The model under review builds one solid part; all positions refer to its coordinate system, in mm. A direction names the side the tool comes from. Coordinates: 2 decimals unless noted, no trailing zeros. Loops run counter-clockwise (first coordinate to the right, second up) from the corner with the lowest first, then second, coordinate; pieces in that order, holes last. Notation, with made-up numbers: M -27,-24.5 L 12,-24.5 A22 ccw 12,-14.5 Z; hole C 76,4.25 d7. An arc over 180 degrees is marked long. Use CSV: the item, a comma, the result in double quotes. Start each with the question number.
from build123d import *

# Parameters (mm, degrees)
SKETCH1_R           = 2.286
SKETCH1_R_2         = 1.27
BOSS_EXTRUDE1_DEPTH = 3.048
BOSS_EXTRUDE2_START = -3.048
BOSS_EXTRUDE2_DEPTH = 3.048
CIRPATTERN2_COUNT   = 18
BOSS_EXTRUDE3_START = 2.54
SKETCH3_R           = 1.75
SKETCH3_R_2         = 1.27
BOSS_EXTRUDE3_DEPTH = 2.54


with BuildPart() as part:
    # Sketch1 → Boss-Extrude1 (new body)
    with BuildSketch(Plane(origin=(0, 0, 0), x_dir=(1, 0, 0), z_dir=(0, 1, 0))):
        with Locations(Location((0, 0, 0), (0, 0, 90))):
            Circle(SKETCH1_R)
        with Locations(Location((0, 0, 0), (0, 0, 90))):
            Circle(SKETCH1_R_2, mode=Mode.SUBTRACT)
    extrude(amount=BOSS_EXTRUDE1_DEPTH)

    # Sketch2 → Boss-Extrude2 (add)
    with BuildSketch(Plane(origin=(0, 3.048, 0), x_dir=(1, 0, 0), z_dir=(0, 1, 0)).offset(BOSS_EXTRUDE2_START)):
        with BuildLine():
            Line((-0.127, 2.794), (0.127, 2.794))
            Line((0.127, 2.794), (0.381, 2.254026397))
            ThreePointArc((0.381, 2.254026397), (0, 2.286), (-0.381, 2.254026397))
            Line((-0.381, 2.254026397), (-0.127, 2.794))
        make_face()
    boss_extrude2 = extrude(amount=BOSS_EXTRUDE2_DEPTH)

    # CirPattern2: Boss-Extrude2 ×18 about axis
    cirpattern2_axis = Axis((0, 0, 0), (0, 1, 0))
    for i in range(1, CIRPATTERN2_COUNT):
        add(boss_extrude2.rotate(cirpattern2_axis, i * 360 / CIRPATTERN2_COUNT))

    # Sketch3 → Boss-Extrude3 (add)
    with BuildSketch(Plane(origin=(0, 0, 0), x_dir=(-1, 0, 0), z_dir=(0, -1, 0)).offset(BOSS_EXTRUDE3_START)):
        with Locations(Location((0, 0, 0), (0, 0, 270))):
            Circle(SKETCH3_R)
        with Locations(Location((0, 0, 0), (0, 0, 90))):
            Circle(SKETCH3_R_2, mode=Mode.SUBTRACT)
    extrude(amount=-BOSS_EXTRUDE3_DEPTH)


solid = part.part
1. To check wall thickness, follow line 1 along X through (y, z) = (-1.5, 0); line 2 along Z through (x, y) = (0, 1.65); line 3 along X through (y, z) = (1, -2.15). State the ranges of each line that lie inside material, in increasing order.
2. For faces 1 (the flat face through (-2, 0, 0)), 2 (the flat face through (-0.6, 3.048, -1.3)), list the 3-axis set-ups (+Z, -Z, +X, -X, +Y, -Y) from which the entire face can be reached by the end or side of a thin tool; tool diameter is ignored.
3. Add section C-C (y = -1.7). Write out the cut boundary in (x, z).
4. Add section A-A (x = 0). Write out the cut boundary in (y, z), plus the area to 3 significant figures.
5. Add section B-B (z = -0.1). Write out the cut boundary in (x, y).
6. Add section D-D (x = 1.45). Write out the cut boundary in (y, z), plus the area to 3 significant figures.
Solved:
1,line 1,"x = -1.75 to -1.27, 1.27 to 1.75"
1,line 2,"z = -2.79 to -1.27, 1.27 to 2.79"
1,line 3,"x = -1.78 to -1.54, -1.11 to 1.11, 1.54 to 1.78"
2,face 1,"-Y"
2,face 2,"+Z, -Z, +X, -X, +Y"
3,outline,"C 0,0 d3.5; hole C 0,0 d2.54"
4,outline,"M -2.54,-1.75 L 0,-1.75 L 0,-2.79 L 3.05,-2.79 L 3.05,-1.27 L -2.54,-1.27 Z; M -2.54,1.27 L 3.05,1.27 L 3.05,2.79 L 0,2.79 L 0,1.75 L -2.54,1.75 Z"
4,area,"11.7 mm^2"
5,outline,"M -2.4,0 L -1.75,0 L -1.75,-2.54 L -1.27,-2.54 L -1.27,3.05 L -2.4,3.05 Z; M 1.27,-2.54 L 1.75,-2.54 L 1.75,0 L 2.4,0 L 2.4,3.05 L 1.27,3.05 Z"
6,outline,"M -2.54,-0.98 L 0,-0.98 L 0,-2.11 L 3.05,-2.11 L 3.05,2.11 L 0,2.11 L 0,0.98 L -2.54,0.98 Z"
6,area,"17.8 mm^2"
